Could you check a few things on this model? Use its own coordinates, in mm. Face numbers are marked on the shaded views. A direction names the side the tool comes from. Give positions to 0.01 mm unless a question says otherwise; leave off trailing zeros. Loops run counter-clockwise (first coordinate to the right, second up) from the corner with the lowest first, then second, coordinate; pieces in that order, holes last. Notation, with made-up numbers: M 2.5,6 L 15.5,6 A17 cw 15.5,29 Z; hole C -19,19 d11. An arc over 180 degrees is marked long. Return JSON: item names as keys, results as strings. Group by question number.
1. For the marked faces 1, 2, 3, 4 and 5, which set-ups out of +Z, -Z, +X, -X, +Y, -Y let a thin tool reach every point of the face, with its end or its side?
2. Please list where these lines run through material, in increasing order: line 1 (Z direction, x = 20, y = 16) (3 decimals); line 2 (X direction, y = 5, z = 12.5) (3 decimals); line 3 (Z direction, x = 85.5, y = -4.5) (3 decimals).
3. For pin 1 (10 mm diameter, centred on x = 44.5, z = 36.5, fed in from -Y); pin 2 (8 mm diameter, centred on x = 7.5, z = 51, fed in from +Y) (3 decimals); pin 3 (14 mm diameter, centred on y = -15, z = 21, fed in from -X) (3 decimals), each with a flat end and sliding along its axis, tell me the tip position at first contact or that it passes through.
4. If we section it at A-A (y = -22.5): Write out the boundary of the cut face in (x, z) (3 decimals), plus the area to 3 significant figures.
5. If we section it at D-D (y = 5): Write out the boundary of the cut face in (x, z) (3 decimals), plus the area to 3 significant figures.
6. If we section it at C-C (x = 98.5): Write out the boundary of the cut face in (y, z) (3 decimals), plus the area to 3 significant figures.
7. If we section it at B-B (z = 3): Write out the boundary of the cut face in (x, y) (3 decimals), plus the area to 3 significant figures.
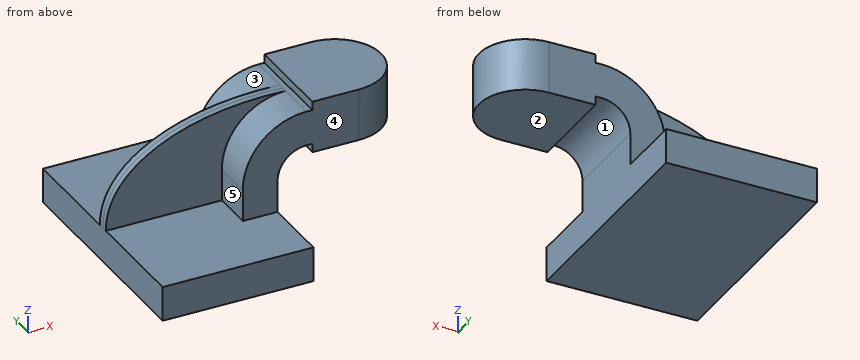
```python
from build123d import *

# Parameters (mm, degrees)
F1_DEPTH = 63.5
F0_W     = 25.4
F0_H     = 19.05
F0_H_2   = 4.7498
F0_H_3   = 4.7752
F2_DEPTH = 25.4
F3_DEPTH = 3.175


with BuildPart() as f1:
    # F0 (on Front) → F1 (new body, symmetric)
    with BuildSketch(Plane.XZ):
        Polygon((-41.275, -9.525), (41.275, -9.525), (41.275, 9.525), (22.225, 9.525), (-41.275, 9.525), align=None)
    extrude(amount=F1_DEPTH, both=True)

    # F0 (on Front) → F2 (join, symmetric)
    with BuildSketch(Plane.XZ):
        with BuildLine():
            Line((22.225, 9.525), (41.275, 9.525))
            Line((41.275, 9.525), (41.275, 27.0002))
            ThreePointArc((41.275, 27.0002), (45.9246798487, 38.2255201513), (57.15, 42.8752))
            Line((57.15, 42.8752), (60.325, 42.8752))
            Line((60.325, 42.8752), (60.325, 61.9252))
            Line((60.325, 61.9252), (57.15, 61.9252))
            ThreePointArc((57.15, 61.9252), (32.4542956671, 51.6959043329), (22.225, 27.0002))
            Line((22.225, 27.0002), (22.225, 9.525))
        make_face()
        with Locations((73.025, 52.4002)):
            Rectangle(F0_W, F0_H)
        with Locations((73.025, 64.3001)):
            Rectangle(F0_W, F0_H_2)
        with Locations((73.025, 40.4876)):
            Rectangle(F0_W, F0_H_3)
    extrude(amount=F2_DEPTH, both=True)

    # F0 (on Front) → F3 (join, symmetric)
    with BuildSketch(Plane.XZ):
        with BuildLine():
            add(Edge.make_bspline(
                [(-41.275, 9.525), (-41.6004359722, 42.6694862545), (0, 64.4797682762), (57.15, 61.9252)],
                knots=[0, 0, 0, 0, 111.5045361635, 111.5045361635, 111.5045361635, 111.5045361635], degree=3))
            Line((-41.275, 9.525), (22.225, 9.525))
            Line((22.225, 9.525), (22.225, 27.0002))
            ThreePointArc((22.225, 27.0002), (32.4542956671, 51.6959043329), (57.15, 61.9252))
        make_face()
    extrude(amount=F3_DEPTH, both=True)

    # F0 (on Front) → F4 (revolve)
    with BuildSketch(Plane.XZ):
        Polygon((85.725, 66.675), (85.725, 61.9252), (85.725, 42.8752), (85.725, 38.1), (111.125, 38.1), (111.125, 66.675), align=None)
    revolve(axis=Axis((85.725, 0, 52.3875), (0, 0, 1)))


solid = f1.part
```
Answer:
{
 "1": {"face 1": "-Z, +Y, -Y", "face 2": "-Z, +X, +Y, -Y", "face 3": "+Z, -X, +Y", "face 4": "+Z, +X, -X, -Y", "face 5": "+Z, -X, -Y"},
 "2": {"line 1": "z = -9.525 to 9.525", "line 2": "x = 22.225 to 41.275", "line 3": "z = 38.1 to 66.675"},
 "3": {"pin 1": "stops at y = -25.4", "pin 2": "stops at y = 3.175", "pin 3": "stops at x = 22.225"},
 "4": {"outline": "M -41.275,-9.525 L 41.275,-9.525 L 41.275,27 A15.875 cw 57.15,42.875 L 60.325,42.875 L 60.325,38.1 L 97.511,38.1 L 97.511,66.675 L 60.325,66.675 L 60.325,61.925 L 57.15,61.925 A34.925 ccw 22.225,27 L 22.225,9.525 L -41.275,9.525 Z", "area": "3,790 mm²"},
 "5": {"outline": "M -41.275,-9.525 L 41.275,-9.525 L 41.275,27 A15.875 cw 57.15,42.875 L 60.325,42.875 L 60.325,38.1 L 110.628,38.1 L 110.628,66.675 L 60.325,66.675 L 60.325,61.925 L 57.15,61.925 A34.925 ccw 22.225,27 L 22.225,9.525 L -41.275,9.525 Z", "area": "4,160 mm²"},
 "6": {"outline": "M -21.954,38.1 L 21.954,38.1 L 21.954,66.675 L -21.954,66.675 Z", "area": "1,250 mm²"},
 "7": {"outline": "M -41.275,-63.5 L 41.275,-63.5 L 41.275,63.5 L -41.275,63.5 Z", "area": "10,500 mm²"}
}
